from build123d import *

# Parameters (mm, degrees)
F1_DEPTH = 12.7
F2_COUNT = 8
F3_SIZE  = 1.524
F4_R     = 7.62
F5_DEPTH = 0.889
F6_W     = 6.4008
F6_H     = 6.4008
F7_DEPTH = 3.81
F8_R     = 3.0988
F9_DEPTH = 8.002


with BuildPart() as f1:
    # F0 (on Front) → F1 (new body)
    with BuildSketch(Plane.XZ):
        with BuildLine():
            Line((0, 0), (0, 15.5699663264))
            ThreePointArc((0, 15.5699663264), (-3.7012650727, 18.6075160708), (-5.9583681556, 14.3847732109))
            ThreePointArc((-5.9583681556, 14.3847732109), (-7.0990438342, 10.6244696981), (-11.00962894, 11.00962894))
            Line((-11.00962894, 11.00962894), (0, 0))
        make_face()
    extrude(amount=F1_DEPTH)

    # F2: F1 ×8 about axis
    f2_axis = Axis((0, -6.35, 0), (0, 1, 0))


with BuildPart() as f1_1:
    add(f1.part)
    for i in range(1, F2_COUNT):
        add(f1.part.rotate(f2_axis, i * 360 / F2_COUNT))

    # F3
    f3_edges = [f1_1.edges().sort_by_distance(p)[0] for p in [
        (-3.701265, -12.7, 18.607516),
    ]]
    chamfer(f3_edges, length=F3_SIZE)

    # F4 (on face) → F5 (cut)
    with BuildSketch(Plane.XZ.offset(12.7)):
        Circle(F4_R)
    extrude(amount=-F5_DEPTH, mode=Mode.SUBTRACT)

    # F6 (on face) → F7 (cut)
    with BuildSketch(Plane.XZ.offset(11.811)):
        Rectangle(F6_W, F6_H)
    extrude(amount=-F7_DEPTH, mode=Mode.SUBTRACT)

    # F8 (on face) → F9 (cut, through all)
    with BuildSketch(Plane.XZ.offset(8.001)):
        Circle(F8_R)
    extrude(amount=-F9_DEPTH, mode=Mode.SUBTRACT)


solid = f1_1.part
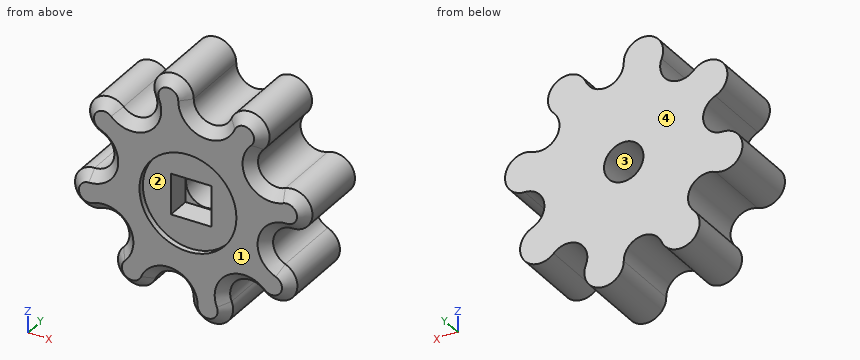
Here's how the part is built. I have some questions about the finished solid (model axes, mm). Face numbers are marked on the shaded views. A direction names the side the tool comes from. Coordinates: 2 decimals unless noted, no trailing zeros. Write each loop counter-clockwise with the first axis right and the second up, starting at its lowest first coordinate (ties: lowest second). Pieces come first, ordered by that corner, then holes.
1) Thinking about a two-plate mould opening in Z: for the marked faces 3 and 4, which applies, +Z half, -Z half, draft (parallel to the pull), parting line (faces both ways), or undercut?
Filled in:
face 3: undercut
face 4: draft
2) If I drill on line 1 (Y direction, x = -5, z = -3); line 2 (Z direction, x = -11.5, y = -5); line 3 (X direction, y = -10.75, z = -13.5), over which ranges is the centre line in solid material (lowest first)?
Filled in:
line 1: y = -11.81 to 0
line 2: z = -14.75 to -11.65, -6.23 to 11.41
line 3: x = -11.9 to -5.4, -0.79 to 5.74
3) Which directions (+Z, -Z, +X, -X, +Y, -Y) give clear straight access to the entire face, cutting with the end or side of a thin tool? Please do the marked faces 1 and 2.
Filled in:
face 1: +Z, -Z, +X, -X, -Y
face 2: -Y
4) If we section it at B-B (y = -9.25): List the corners of the cut face in (x, z) for me.
Filled in:
outline: (-15.57, 0) arc R3.1 ccw (long way) to (-14.38, -5.96) arc R3.1 cw to (-11.01, -11.01) arc R3.1 ccw (long way) to (-5.96, -14.38) arc R3.1 cw to (0, -15.57) arc R3.1 ccw (long way) to (5.96, -14.38) arc R3.1 cw to (11.01, -11.01) arc R3.1 ccw (long way) to (14.38, -5.96) arc R3.1 cw to (15.57, 0) arc R3.1 ccw (long way) to (14.38, 5.96) arc R3.1 cw to (11.01, 11.01) arc R3.1 ccw (long way) to (5.96, 14.38) arc R3.1 cw to (0, 15.57) arc R3.1 ccw (long way) to (-5.96, 14.38) arc R3.1 cw to (-11.01, 11.01) arc R3.1 ccw (long way) to (-14.38, 5.96) arc R3.1 cw to start; hole (-3.2, -3.2) - (3.2, -3.2) - (3.2, 3.2) - (-3.2, 3.2) - close
5) If we section it at A-A (y = -1.5): List the corners of the cut face in (x, z) for me.
Filled in:
outline: (-15.57, 0) arc R3.1 ccw (long way) to (-14.38, -5.96) arc R3.1 cw to (-11.01, -11.01) arc R3.1 ccw (long way) to (-5.96, -14.38) arc R3.1 cw to (0, -15.57) arc R3.1 ccw (long way) to (5.96, -14.38) arc R3.1 cw to (11.01, -11.01) arc R3.1 ccw (long way) to (14.38, -5.96) arc R3.1 cw to (15.57, 0) arc R3.1 ccw (long way) to (14.38, 5.96) arc R3.1 cw to (11.01, 11.01) arc R3.1 ccw (long way) to (5.96, 14.38) arc R3.1 cw to (0, 15.57) arc R3.1 ccw (long way) to (-5.96, 14.38) arc R3.1 cw to (-11.01, 11.01) arc R3.1 ccw (long way) to (-14.38, 5.96) arc R3.1 cw to start; hole circle Ø6.2 at (0, 0)
6) I'm going to push flat-ended pins straight in: pin 1 (1.1 mm diameter, centred on y = -11, z = 0, fed in from -X); pin 2 (5 mm diameter, centred on x = -9.5, z = 13.5, fed in from +Y); pin 3 (1 mm diameter, centred on y = -3, z = 7, fed in from -X); pin 4 (7.5 mm diameter, centred on x = -2, z = -2, fed in from -Y). Where does each tip first touch, or does it pass through?
Filled in:
pin 1: stops at x = -17.33
pin 2: passes through
pin 3: stops at x = -16
pin 4: stops at y = -11.81
